Part model, mm, in its own coordinate system. A direction names the side the tool comes from. Coordinates: 2 decimals unless noted, no trailing zeros. Write each loop counter-clockwise with the first axis right and the second up, starting at its lowest first coordinate (ties: lowest second). Pieces come first, ordered by that corner, then holes. Notation, with made-up numbers: (-25, 8) - (-6, 8) arc R9 ccw to (-6, 19) - close; hole circle Ø4 at (17, 36.25). An arc over 180 degrees is marked (long way). Use a Markdown table: item, result.
```python
from build123d import *

# Parameters (mm, degrees)
SKETCH_1_W               = 16
SKETCH_1_H               = 8.2
EXTRUDE_1_DEPTH          = 10.3
EXTRUDE_START            = 10.3
SKETCH_2_W               = 23
SKETCH_2_H               = 8.2
EXTRUDE_2_DEPTH          = 1
SKETCH_3_W               = 16
SKETCH_3_H               = 8.2
EXTRUDE_3_DEPTH          = 14.5
SKETCH_4_R               = 1
CUT_EXTRUDE_1_DEPTH      = 14.5
EXTRUDE_4_DEPTH          = 16.9
SKETCH_7_R               = 1.5
EXTRUDE_5_DEPTH          = 19.9
CUT_EXTRUDE_2_DEPTH      = 10
CUT_EXTRUDE_2_DEPTH_BACK = 10


with BuildPart() as part:
    # 草图1 → 凸台-拉伸1 (new body)
    with BuildSketch(Plane(origin=(0, 0, 0), x_dir=(1, 0, 0), z_dir=(0, 1, 0))):
        Rectangle(SKETCH_1_W, SKETCH_1_H)
    extrude(amount=EXTRUDE_1_DEPTH)

    # 草图2 → 凸台-拉伸2 (add)
    with BuildSketch(Plane(origin=(0, 0, 0), x_dir=(1, 0, 0), z_dir=(0, 1, 0)).offset(EXTRUDE_START)):
        Rectangle(SKETCH_2_W, SKETCH_2_H)
    extrude(amount=EXTRUDE_2_DEPTH)

    # 草图3 → 凸台-拉伸3 (add)
    with BuildSketch(Plane(origin=(0, 0, 0), x_dir=(1, 0, 0), z_dir=(0, 1, 0))):
        Rectangle(SKETCH_3_W, SKETCH_3_H)
    extrude(amount=EXTRUDE_3_DEPTH)

    # 草图4 → 切除-拉伸1 (cut)
    with BuildSketch(Plane(origin=(0, 0, 0), x_dir=(1, 0, 0), z_dir=(0, 1, 0))):
        with Locations(Location((-9.75, 0, 0), (0, 0, 90))):
            Circle(SKETCH_4_R)
        with Locations(Location((9.75, 0, 0), (0, 0, 90))):
            Circle(SKETCH_4_R)
    extrude(amount=CUT_EXTRUDE_1_DEPTH, mode=Mode.SUBTRACT)

    # 草图6 → 凸台-拉伸4 (add)
    with BuildSketch(Plane(origin=(0, 0, 0), x_dir=(1, 0, 0), z_dir=(0, 1, 0))):
        with BuildLine():
            Line((8, 1.86748494), (8, -1.86748494))
            ThreePointArc((8, -1.86748494), (5.822893402, -3.826301743), (2.894290795, -3.832872384))
            Line((2.894290795, -3.832872384), (-1.8, -2.05))
            ThreePointArc((-1.8, -2.05), (-3.85, 0), (-1.8, 2.05))
            Line((-1.8, 2.05), (2.894290795, 3.832872384))
            ThreePointArc((2.894290795, 3.832872384), (5.822893402, 3.826301743), (8, 1.86748494))
        make_face()
    extrude(amount=EXTRUDE_4_DEPTH)

    # 草图7 → 凸台-拉伸5 (add)
    with BuildSketch(Plane(origin=(0, 0, 0), x_dir=(1, 0, 0), z_dir=(0, 1, 0))):
        with Locations(Location((4.35, 0, 0), (0, 0, 90))):
            Circle(SKETCH_7_R)
    extrude(amount=EXTRUDE_5_DEPTH)

    # 草图8 → 切除-拉伸2 (cut, two sides: drawn at the far end of the back side and taken through both)
    with BuildSketch(Plane.XY.offset(-CUT_EXTRUDE_2_DEPTH_BACK)):
        Polygon((-8, 14.5), (-8, 13.5), (-4.85, 14.5), align=None)
    extrude(amount=CUT_EXTRUDE_2_DEPTH + CUT_EXTRUDE_2_DEPTH_BACK, mode=Mode.SUBTRACT)


solid = part.part
```
Item 1: Drop flat-ended pins along their axis: P1, Ø1.1, axis at x = 5.5, z = 2.5, coming from the +Y side; P2, Ø4.5, axis at y = 14, z = 2, coming from the +X side; P3, Ø1.8, axis at x = -9, z = 1, coming from the +Y side. Give the stop position or say it passes through.
From the geometry:
| item | result |
|---|---|
| P1 | y = 16.9 |
| P2 | x = 8 |
| P3 | y = 11.3 |
Item 2: Which spindle directions (+Z, -Z, +X, -X, +Y, -Y) get a long thin tool onto all of the face, cutting with end or side? Do faces 1 (the face through (-4.4, 14.5, -0.1)), 2 (the face through (-9, 10.3, -1)), 3 (the face through (8, 13, 0)). Say none if no direction does.
From the geometry:
| item | result |
|---|---|
| face 1 | -X, +Y |
| face 2 | +Z, -Z, -X, -Y |
| face 3 | +Z, -Z, +X, +Y |
Item 3: Band-saw the part on B-B, the plane z = 0. Give the cut face in (x, y), then the cut area to 3 significant figures.
From the geometry:
| item | result |
|---|---|
| outline | (-11.5, 10.3) - (-10.75, 10.3) - (-10.75, 11.3) - (-11.5, 11.3) - close; (-8.75, 10.3) - (-8, 10.3) - (-8, 0) - (8, 0) - (8, 10.3) - (8.75, 10.3) - (8.75, 11.3) - (8, 11.3) - (8, 16.9) - (5.85, 16.9) - (5.85, 19.9) - (2.85, 19.9) - (2.85, 16.9) - (-3.85, 16.9) - (-3.85, 14.5) - (-4.85, 14.5) - (-8, 13.5) - (-8, 11.3) - (-8.75, 11.3) - close; (10.75, 10.3) - (11.5, 10.3) - (11.5, 11.3) - (10.75, 11.3) - close |
| area | 271 mm^2 |
Item 4: Drill centre lines: probe 1 along X at (y, z) = (11.1, 0); probe 2 along X at (y, z) = (5, -3); probe 3 along Y at (x, z) = (0, 2.25). Where is each one in solid material? Low to high.
From the geometry:
| item | result |
|---|---|
| probe 1 | -11.5 to -10.75, -8.75 to 8.75, 10.75 to 11.5 |
| probe 2 | -8 to 8 |
| probe 3 | 0 to 16.9 |
Item 5: Band-saw the part on D-D, the plane y = 11. Give the cut face in (x, z).
From the geometry:
| item | result |
|---|---|
| outline | (-11.5, -4.1) - (11.5, -4.1) - (11.5, 4.1) - (-11.5, 4.1) - close; hole circle Ø2 at (-9.75, 0); hole circle Ø2 at (9.75, 0) |
Item 6: Band-saw the part on A-A, the plane x = 9.75. Give the cut face in (y, z), then the cut area to 3 significant figures.
From the geometry:
| item | result |
|---|---|
| outline | (10.3, -4.1) - (11.3, -4.1) - (11.3, -1) - (10.3, -1) - close; (10.3, 1) - (11.3, 1) - (11.3, 4.1) - (10.3, 4.1) - close |
| area | 6.20 mm^2 |
Item 7: Band-saw the part on C-C, the plane x = 5.25. Give the cut face in (y, z).
From the geometry:
| item | result |
|---|---|
| outline | (0, -4.1) - (14.5, -4.1) - (14.5, -4) - (16.9, -4) - (16.9, -1.2) - (19.9, -1.2) - (19.9, 1.2) - (16.9, 1.2) - (16.9, 4) - (14.5, 4) - (14.5, 4.1) - (0, 4.1) - close |
Item 8: Two-plate mould, pull along X, no slides. Class faces 4 (the face through (8, 5, 0)), 5 (the face through (-10.74, 10.79, 0.13)), 6 (the face through (4, 19.9, 0)): pulls with the +X half, pulls with the -X half, needs draft (parallel to the pull), parting line crosses it, or undercut.
From the geometry:
| item | result |
|---|---|
| face 4 | pulls with the +X half |
| face 5 | undercut |
| face 6 | needs draft |
